Could you check a few things on this model? Use its own coordinates, in mm. Face numbers are marked on the shaded views. Give positions to 0.01 mm unless a question says otherwise; leave off trailing zeros. Loops run counter-clockwise (first coordinate to the right, second up) from the corner with the lowest first, then second, coordinate; pieces in that order, holes last. Notation, with made-up numbers: (-27.75, -16) - (14.25, -16) arc R24 cw to (14.25, 22) - close; hole circle Ø1 at (46, 3.25). An arc over 180 degrees is marked (long way). Write each question's results on one line, items separated by ' | '. Start each with the question number.
Solid Edge part; units mm, degrees
sketch "Sketch1" plane through (0, 0, 0) normal (0, -1, 0) x (1, 0, 0)
  circle A0 centre (0, 0) radius 9
extrude "Ajout_matière_1" add sketch "Sketch1" against normal blind 3
sketch "Sketch2" plane through (0, 3, 0) normal (0, 1, 0) x (-1, 0, 0)
  circle A0 centre (0, -7) radius 1.075
  circle A1 centre (0, 0) radius 1.5
  circle A2 centre (0, 7) radius 1.075
extrude "Enlèvement_matière_1" cut sketch "Sketch2" against normal blind 8.787
chamfer "Chamfer1" distance 1 angle 45 1 edges at (1.5, 3, 0)
properties part number "14" material "PMMA"
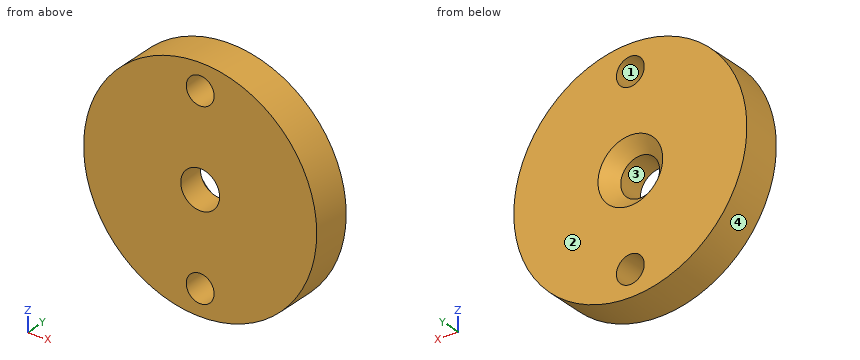
Q1. I want a section at D-D, the plane z = 7.5. List the corners of the cut face in (x, y) for me.
Q2. I want a section at B-B, the plane z = 0. List the corners of the cut face in (x, y) for me, then the cut area to 3 significant figures.
Q3. If we mould it in two halves opening along Z, with no side actions, what happens to the marked faces 1, 2, 3 and 4? For each: +Z half, -Z half, draft (parallel to the pull), parting line (faces both ways), or undercut.
Q4. I want a section at C-C, the plane y = 1.7. List the corners of the cut face in (x, z) for me (3 decimals).
Q5. I want a section at A-A, the plane x = 0. List the corners of the cut face in (y, z) for me (3 decimals).
Q6. I'm going to push flat-ended pins straight in: pin 1 Ø1 at (x, y) = (3, 2) entering from -Z; pin 2 Ø1.5 at (x, y) = (-6, 1) entering from -Z; pin 3 Ø4 at (x, z) = (0, 0) entering from +Y. Where does each tip first touch, or does it pass through?
Q7. I need wall thicknesses on L1, parallel to Z at x = 0, y = 1.3 (3 decimals); L2, parallel to Z at x = 0, y = 2.1 (3 decimals); L3, parallel to X at y = 1.45, z = 6.75. Which ranges of each line are inside material? Lowest first, please. Write a range as from..to.
Conclusion:
1) outline: (-4.97, 0) - (-0.95, 0) - (-0.95, 3) - (-4.97, 3) - close; (0.95, 0) - (4.97, 0) - (4.97, 3) - (0.95, 3) - close
2) outline: (-9, 0) - (-1.5, 0) - (-1.5, 2) - (-2.5, 3) - (-9, 3) - close; (1.5, 0) - (9, 0) - (9, 3) - (2.5, 3) - (1.5, 2) - close | area: 44.0 mm^2
3) face 1: undercut | face 2: draft | face 3: undercut | face 4: parting line
4) outline: circle Ø18 at (0, 0); hole circle Ø3 at (0, 0); hole circle Ø2.15 at (0, -7); hole circle Ø2.15 at (0, 7)
5) outline: (0, -9) - (3, -9) - (3, -8.075) - (0, -8.075) - close; (0, -5.925) - (3, -5.925) - (3, -2.5) - (2, -1.5) - (0, -1.5) - close; (0, 1.5) - (2, 1.5) - (3, 2.5) - (3, 5.925) - (0, 5.925) - close; (0, 8.075) - (3, 8.075) - (3, 9) - (0, 9) - close
6) pin 1: z = -8.65 | pin 2: z = -7.31 | pin 3: y = 2.5
7) L1: -9..-8.075, -5.925..-1.5, 1.5..5.925, 8.075..9 | L2: -9..-8.075, -5.925..-1.6, 1.6..5.925, 8.075..9 | L3: -5.95..-1.05, 1.05..5.95
